Check sheet for the modelled part. Datum: model origin and axes. Units: mm. A direction names the side the tool comes from. Coordinates: 2 decimals unless noted, no trailing zeros. Loops run counter-clockwise (first coordinate to the right, second up) from the corner with the lowest first, then second, coordinate; pieces in that order, holes last. Notation, with made-up numbers: (82, 31.25) -> (89, 31.25) arc R35 cw to (89, 65.25) -> close; hole circle Ø6 at (39.25, 76.25). An arc over 180 degrees is marked (long way). Use CSV: the item, a comma, the result in double quotes.
Autodesk Inventor part; units mm, degrees
ref_plane "YZ Plane" through (0, 0, 0) normal (1, 0, 0) x (0, 1, 0)
ref_plane "XZ Plane" through (0, 0, 0) normal (0, 1, 0) x (-1, 0, 0)
ref_plane "XY Plane" through (0, 0, 0) normal (0, 0, 1) x (1, 0, 0)
sketch "Sketch1" plane through (0, 0, 0) normal (0, 0, 1) x (1, 0, 0)
  circle A0 centre (0, 0) radius 5.0165
  dimension "d0" = 10.033
extrude "Extrusion1" add sketch "Sketch1" against normal blind 1.27
sketch "Sketch2" plane through (0, 0, -1.27) normal (0, 0, -1) x (-1, 0, 0)
  circle A0 centre (0, 0) radius 5.0165
  line L0 (-3.1496, -3.1496) -> (3.1496, -3.1496)
  line L1 (3.1496, -3.1496) -> (3.1496, 3.1496)
  line L2 (3.1496, 3.1496) -> (-3.1496, 3.1496)
  line L3 (-3.1496, 3.1496) -> (-3.1496, -3.1496)
  point P0 (0, 3.1496)
  point P1 (-3.1496, 0)
  dimension "d3" = 6.2992
extrude "Extrusion2" add sketch "Sketch2" along normal blind 3.81 contours L3 L2 L1 L0
fillet "Fillet1" radius 0.508 8 edges at (3.1496, 3.1496, -3.175) (-3.1496, 3.1496, -3.175) (-3.1496, -3.1496, -3.175) (3.1496, -3.1496, -3.175) (3.1496, 0, -5.08) (0, 3.1496, -5.08) (-3.1496, 0, -5.08) (0, -3.1496, -5.08)
sketch "Sketch4" plane through (0, 0, 0) normal (0, 0, 1) x (1, 0, 0)
  circle A0 centre (0, 0) radius 5.0165
  line L0 (-1.5875, -1.5875) -> (1.5875, -1.5875)
  line L1 (1.5875, -1.5875) -> (1.5875, 1.5875)
  line L2 (1.5875, 1.5875) -> (-1.5875, 1.5875)
  line L3 (-1.5875, 1.5875) -> (-1.5875, -1.5875)
  point P0 (0, 1.5875)
  point P1 (-1.5875, 0)
  dimension "d14" = 3.175
extrude "Extrusion3" cut sketch "Sketch4" against normal through all contours L3 L2 L1 L0
fillet "Fillet2" radius 0.254 4 edges at (-1.5875, 1.5875, -2.54) (1.5875, 1.5875, -2.54) (-1.5875, -1.5875, -2.54) (1.5875, -1.5875, -2.54)
sketch "Sketch5" plane through (0, 0, 0) normal (0, 0, 1) x (1, 0, 0)
  line L0 (-1.3335, 1.5875) -> (1.3335, 1.5875)
  circle A0 centre (0, 0) radius 5.0165
  circle A1 centre (0, 0) radius 1.5875
surface extrude "ExtrusionSrf1" sketch "Sketch5" against normal up to surface (5.08 mm away) shown no curves A1
properties part number "High Strength Square Gear Insert" material "Acetal Resin, White"
1) Access from +Z, -Z, +X, -X, +Y, -Y to the whole of each face (thin tool, end or side, straight path). Record for faces 1 (the flat face through (-3.15, 0, -3)), 2 (the flat face through (1.588, 0, -3)), 3 (the flat face through (0, 3.15, -3)), 4 (the flat face through (-0.1, -3.3, -1.27)).
Answer below:
face 1,"-Z, -X, +Y, -Y"
face 2,"+Z, -Z"
face 3,"-Z, +X, -X, +Y"
face 4,"-Z"
2) Cross-section at C-C on z = -0.5. Record the boundary of the cut face in (x, y).
Answer below:
outline,"circle Ø10.03 at (0, 0); hole (-1.59, -1.33) arc R0.25 ccw to (-1.33, -1.59) -> (1.33, -1.59) arc R0.25 ccw to (1.59, -1.33) -> (1.59, 1.33) arc R0.25 ccw to (1.33, 1.59) -> (-1.33, 1.59) arc R0.25 ccw to (-1.59, 1.33) -> close"
3) Cross-section at A-A on x = 0. Record the boundary of the cut face in (y, z).
Answer below:
outline,"(-5.02, -1.27) -> (-3.15, -1.27) -> (-3.15, -4.57) arc R0.51 ccw to (-2.64, -5.08) -> (-1.59, -5.08) -> (-1.59, 0) -> (-5.02, 0) -> close; (1.59, -5.08) -> (2.64, -5.08) arc R0.51 ccw to (3.15, -4.57) -> (3.15, -1.27) -> (5.02, -1.27) -> (5.02, 0) -> (1.59, 0) -> close"
4) Cross-section at D-D on z = -1.4. Record the boundary of the cut face in (x, y), and give its area (3 significant figures).
Answer below:
outline,"(-3.15, -2.64) arc R0.51 ccw to (-2.64, -3.15) -> (2.64, -3.15) arc R0.51 ccw to (3.15, -2.64) -> (3.15, 2.64) arc R0.51 ccw to (2.64, 3.15) -> (-2.64, 3.15) arc R0.51 ccw to (-3.15, 2.64) -> close; hole (-1.59, -1.33) arc R0.25 ccw to (-1.33, -1.59) -> (1.33, -1.59) arc R0.25 ccw to (1.59, -1.33) -> (1.59, 1.33) arc R0.25 ccw to (1.33, 1.59) -> (-1.33, 1.59) arc R0.25 ccw to (-1.59, 1.33) -> close"
area,"29.4 mm²"
5) Draft check along X on faces 5 (the flat face through (3.15, 0, -3)), 6 (the flat face through (-1.588, 0, -3)), 7 (the flat face through (0, -3.15, -3)). Enter one of: released by +X, released by -X, zero draft, split by the parting line, or undercut.
Answer below:
face 5,"released by +X"
face 6,"undercut"
face 7,"zero draft"
6) Thickness scan on line 1 along Y through (x, z) = (-1, -3.05); line 2 along X through (y, z) = (2.25, -3.4). Record the ranges inside material, lowest first. Write a range as from..to.
Answer below:
line 1,"y = -3.15..-1.59, 1.59..3.15"
line 2,"x = -3.15..3.15"
7) Go/stop test with flat-tipped pins: pin 1 Ø2.5 at (x, z) = (0, -2) entering from -Y; pin 2 Ø0.8 at (y, z) = (0.5, -1.5) entering from +X; pin 3 Ø1 at (y, z) = (0, -3) entering from -X; pin 4 Ø2 at (y, z) = (-3.5, -1) entering from +X. Record where each tip stops, or that it passes through.
Answer below:
pin 1,"stops at y = -5.02"
pin 2,"stops at x = 5.01"
pin 3,"stops at x = -3.15"
pin 4,"stops at x = 4.35"
